from build123d import *

# Parameters (mm, degrees)
F0_R     = 4
F1_DEPTH = 6
F2_R     = 5
F3_R     = 1


with BuildPart() as f1:
    # F0 (on Front) → F1 (new body)
    with BuildSketch(Plane.XZ):
        with BuildLine():
            Line((40.613971, 0), (-40.666029, 0))
            Line((-40.666029, 0), (-43.802427, -5.227331))
            Line((-43.802427, -5.227331), (18.873971, -25.4))
            ThreePointArc((18.873971, -25.4), (25.373971, -18.9), (31.873971, -25.4))
            Line((31.873971, -25.4), (35.371493, -25.4))
            Line((35.371493, -25.4), (40.613971, -25.4))
            Line((40.613971, -25.4), (40.613971, -10.16))
            Line((40.613971, -10.16), (40.613971, -7.62))
            Line((40.613971, -7.62), (40.613971, -6.35))
            Line((40.613971, -6.35), (40.613971, 0))
        make_face()
        with Locations((-10.186029, -7.62)):
            Circle(F0_R, mode=Mode.SUBTRACT)
        with Locations((15.213971, -10.16)):
            Circle(F0_R, mode=Mode.SUBTRACT)
    extrude(amount=F1_DEPTH)

    # F2
    f2_edges = [f1.edges().sort_by_distance(p)[0] for p in [
        (40.613971, -3, 0),
    ]]
    fillet(f2_edges, radius=F2_R)

    # F3
    f3_edges = [f1.edges().sort_by_distance(p)[0] for p in [
        (31.873971, -3, -25.4),
    ]]
    fillet(f3_edges, radius=F3_R)


solid = f1.part
Model file for the job. Use its own axes, mm. Give positions to 0.01 mm unless a question says otherwise; leave off trailing zeros. Order: outer loops, then holes, each group sorted by start corner. A loop starts at its lowest first (then second) coordinate and runs counter-clockwise, first axis right, second up. Notation, with made-up numbers: (64, -36) -> (111, -36) arc R19 cw to (111, -7) -> close; hole circle Ø10 at (16.25, 75.25). An arc over 180 degrees is marked (long way). Use CSV: the item, a comma, the result in double quotes.
1. Drill centre lines: line 1 along Z through (x, y) = (15, -5.35); line 2 along Z through (x, y) = (-13.5, -4.6); line 3 along Z through (x, y) = (-32.5, -1.25). Where is each one in solid material? Low to high. Write a range as from..to.
Outcome:
line 1,"-24.15..-14.15, -6.17..0"
line 2,"-14.98..-9.86, -5.38..0"
line 3,"-8.87..0"
2. Band-saw the part on B-B, the plane z = -7.62. Give the cut face in (x, y), then the cut area to 3 significant figures.
Outcome:
outline,"(-36.37, -6) -> (-14.19, -6) -> (-14.19, 0) -> (-36.37, 0) -> close; (-6.19, -6) -> (12.12, -6) -> (12.12, 0) -> (-6.19, 0) -> close; (18.3, -6) -> (40.61, -6) -> (40.61, 0) -> (18.3, 0) -> close"
area,"377 mm²"
3. Band-saw the part on A-A, the plane y = -3. Give the cut face in (x, z).
Outcome:
outline,"(-43.8, -5.23) -> (18.87, -25.4) arc R6.5 cw to (31.82, -24.53) arc R1 ccw to (32.81, -25.4) -> (40.61, -25.4) -> (40.61, -5) arc R5 ccw to (35.61, 0) -> (-40.67, 0) -> close; hole circle Ø8 at (-10.19, -7.62); hole circle Ø8 at (15.21, -10.16)"
4. Mould opens along X. For faces 1 (the flat face through (-2, -3, 0)), 2 (the cylindrical face through (17.06, -2.96, -13.71)), 3 (the flat face through (-12.903, -2.958, -15.172)) say: +X half, -X half, draft (parallel to the pull), parting line (faces both ways), or undercut.
Outcome:
face 1,"draft"
face 2,"undercut"
face 3,"-X half"
5. Drop a flat-ended pin along its axis: pin 1 (3 mm diameter, centred on y = -4.5, z = -5.5, fed in from -X). Give the stop position or say it passes through.
Outcome:
pin 1,"x = -43.8"
6. Band-saw the part on C-C, the plane x = 17. Give the cut face in (y, z), then the cut area to 3 significant figures.
Outcome:
outline,"(-6, -24.8) -> (0, -24.8) -> (0, -13.74) -> (-6, -13.74) -> close; (-6, -6.58) -> (0, -6.58) -> (0, 0) -> (-6, 0) -> close"
area,"106 mm²"
7. Band-saw the part on D-D, the plane z = -21.5. Give the cut face in (x, y), then the cut area to 3 significant figures.
Outcome:
outline,"(6.76, -6) -> (20.17, -6) -> (20.17, 0) -> (6.76, 0) -> close; (30.57, -6) -> (40.61, -6) -> (40.61, 0) -> (30.57, 0) -> close"
area,"141 mm²"
